Input: part model. Units: mm. Frame: model coordinates. A direction names the side the tool comes from. Coordinates: 2 decimals unless noted, no trailing zeros. Order: outer loops, then holes, each group sorted by start corner. A loop starts at its lowest first (then second) coordinate and runs counter-clockwise, first axis right, second up. Notation, with made-up numbers: M 11,-8 L 43,-8 A24 cw 43,9 Z; hole C 23.5,-34 d4. An arc over 180 degrees is marked long. One line per item, written item: value.
```python
from build123d import *

# Parameters (mm, degrees)
F0_W      = 95.25
F0_H      = 76.2
F0_R      = 24.665224
F1_DEPTH  = 25.4
F3_R      = 10.074085
F4_DEPTH  = 25.4
F5_R      = 10.419172
F6_DEPTH  = 25.4
F7_R      = 9.130152
F8_DEPTH  = 25.4
F10_R     = 10.023697
F11_DEPTH = 25.4


with BuildPart() as f1:
    # F0 (on Front) → F1 (new body)
    with BuildSketch(Plane.XZ):
        with Locations((-47.625, 2.935028)):
            Rectangle(F0_W, F0_H)
        with Locations((-47.752, 0)):
            Circle(F0_R, mode=Mode.SUBTRACT)
    extrude(amount=F1_DEPTH)

    # F3 (on face) → F4 (cut)
    with BuildSketch(Plane.XY.offset(41.035028)):
        with Locations((-49.393464, -12.561298)):
            Circle(F3_R)
    extrude(amount=-F4_DEPTH, mode=Mode.SUBTRACT)

    # F5 (on face) → F6 (cut)
    with BuildSketch(Plane.YZ):
        with Locations((-12.411524, 0)):
            Circle(F5_R)
    extrude(amount=-F6_DEPTH, mode=Mode.SUBTRACT)

    # F7 (on face) → F8 (cut)
    with BuildSketch(Plane(origin=(-95.25, 0, 0), x_dir=(0, -1, 0), z_dir=(-1, 0, 0))):
        with Locations((10.638449, 0)):
            Circle(F7_R)
    extrude(amount=-F8_DEPTH, mode=Mode.SUBTRACT)

    # F10 (on face) → F11 (cut)
    with BuildSketch(Plane(origin=(0, 0, -35.164972), x_dir=(1, 0, 0), z_dir=(0, 0, -1))):
        with Locations((-51.3951, 13.630712)):
            Circle(F10_R)
    extrude(amount=-F11_DEPTH, mode=Mode.SUBTRACT)


solid = f1.part
```
(1) Cut plane A-A on x = -6.5. Output: boundary loops of the cut face in (y, z), plus the area to 3 significant figures.
Data:
outline: M -25.4,-35.16 L 0,-35.16 L 0,41.04 L -25.4,41.04 Z; hole C -12.41,0 d20.84
area: 1,590 mm2
(2) Ray query, line 1 (Z direction, x = -16.5, y = -12.75); line 2 (X direction, y = -21.25, z = 28.5); line 3 (Z direction, x = -64.5, y = -13.5). Return the intervals inside material, ascending. Write a range as from..to.
Data:
line 1: z = -35.16..-10.41, 10.41..41.04
line 2: x = -95.25..-54.49, -44.3..0
line 3: z = -35.16..-18.11, 18.11..41.04
(3) Cut plane C-C on y = -6.5. Output: boundary loops of the cut face in (x, z).
Data:
outline: M -95.25,-35.16 L -58.44,-35.16 L -58.44,-22.23 A24.67 cw -71.04,-8.14 L -95.25,-8.14 Z; M -95.25,8.14 L -71.04,8.14 A24.67 cw -57.44,22.68 L -57.44,41.04 L -95.25,41.04 Z; M -44.35,-35.16 L 0,-35.16 L 0,-8.58 L -24.63,-8.58 A24.67 cw -44.35,-24.43 Z; M -41.35,23.82 A24.67 cw -24.63,8.58 L 0,8.58 L 0,41.04 L -41.35,41.04 Z
(4) Cut plane D-D on z = -15.5. Output: boundary loops of the cut face in (x, y), plus the area to 3 significant figures.
Data:
outline: M -95.25,-25.4 L -66.94,-25.4 L -66.94,0 L -95.25,0 Z; M -28.57,-25.4 L 0,-25.4 L 0,0 L -28.57,0 Z
area: 1,440 mm2
(5) Access query for faces 5 (the cylindrical face through (-57.39, -18.69, 31.51)), 6 (the cylindrical face through (-61.41, -14.07, -29.58)), 7 (the cylindrical face through (-12.52, -22.82, 0.46)). Directions: +Z, -Z, +X, -X, +Y, -Y. A direction counts if a zero-diameter tool reaches every point of the face in a straight line with its end or side. Return the directions, or none.
Data:
face 5: +Z
face 6: -Z
face 7: +X
(6) Draft query along Z for faces 1 (the cylindrical face through (-83.13, -8.659, -8.913)), 2 (the flat face through (-38, -13, 41.035)), 3 (the cylindrical face through (-36.37, -12.52, -21.88)), 4 (the flat face through (-95.25, -13, 11)). Return one class per face: released by +Z, released by -Z, zero draft, split by the parting line, or undercut.
Data:
face 1: undercut
face 2: released by +Z
face 3: undercut
face 4: zero draft
(7) Cut plane B-B on z = 0. Output: boundary loops of the cut face in (x, y), plus the area to 3 significant figures.
Data:
outline: M -95.25,-25.4 L -72.42,-25.4 L -72.42,-19.77 L -95.25,-19.77 Z; M -95.25,-1.51 L -72.42,-1.51 L -72.42,0 L -95.25,0 Z; M -23.09,-25.4 L 0,-25.4 L 0,-22.83 L -23.09,-22.83 Z; M -23.09,-1.99 L 0,-1.99 L 0,0 L -23.09,0 Z
area: 268 mm2
